from build123d import *

# Parameters (mm, degrees)
F0_W          = 4
F0_H          = 5
F0_R          = 3
F0_W_2        = 2
F0_H_2        = 8
F0_R_2        = 1.2
F1_DEPTH      = 10
F2_DEPTH      = 3
F3_START      = 2
F1_FACE_W     = 45
F1_FACE_H     = 20
F3_DEPTH      = 6.5
F4_START      = 5
F4_DEPTH      = 1.5
F5_R          = 5
F6_DEPTH      = 8.1
F7_DEPTH      = 3
F7_DEPTH_BACK = 0.5
F8_DEPTH      = 25
F8_DEPTH_BACK = 1.7
F10_START     = 16.22
F9_R          = 3.1
F10_DEPTH     = 9.58
F11_START     = 16.7
F9_R_2        = 1.15
F11_DEPTH     = 21.7


with BuildPart() as f1:
    # F0 (on Top) → F1 (new body)
    with BuildSketch(Plane.XY):
        Polygon((21.9938950613, 39.5450913161), (-23.0061049387, 39.5450913161), (-23.0061049387, 19.5450913161), (-9.9312635139, 19.5450913161), (10.0687364861, 19.5450913161), (21.9938950613, 19.5450913161), align=None)
        Polygon((-12.5061049387, 32.0450913161), (-12.5061049387, 37.0450913161), (19.4938950613, 37.0450913161), (19.4938950613, 22.0450913161), (-12.5061049387, 22.0450913161), (-12.5061049387, 27.0450913161), (-16.5061049387, 27.0450913161), (-20.5061049387, 27.0450913161), (-20.5061049387, 32.0450913161), (-16.5061049387, 32.0450913161), align=None, mode=Mode.SUBTRACT)
        with Locations((-18.5061049387, 29.5450913161)):
            Rectangle(F0_W, F0_H)
        with Locations((-14.5061049387, 29.5450913161)):
            Rectangle(F0_W, F0_H)
        Polygon((19.4938950613, 37.0450913161), (-12.5061049387, 37.0450913161), (-12.5061049387, 32.0450913161), (-12.5061049387, 27.0450913161), (-12.5061049387, 22.0450913161), (19.4938950613, 22.0450913161), align=None)
        with Locations((10.4938950613, 30.0450913161)):
            Circle(F0_R, mode=Mode.SUBTRACT)
        with Locations((17.2357911468, 31.5450913161)):
            Rectangle(F0_W_2, F0_H_2, mode=Mode.SUBTRACT)
        with Locations((10.4938950613, 30.0450913161)):
            Circle(F0_R)
        with Locations((10.4938950613, 30.0450913161)):
            Circle(F0_R_2, mode=Mode.SUBTRACT)
        with Locations((10.4938950613, 30.0450913161)):
            Circle(F0_R_2)
        with Locations((17.2357911468, 31.5450913161)):
            Rectangle(F0_W_2, F0_H_2)
    extrude(amount=F1_DEPTH)

    # F0 (on Top) → F2 (join)
    with BuildSketch(Plane.XY):
        Polygon((21.9938950613, 39.5450913161), (-23.0061049387, 39.5450913161), (-23.0061049387, 19.5450913161), (-9.9312635139, 19.5450913161), (10.0687364861, 19.5450913161), (21.9938950613, 19.5450913161), align=None)
        Polygon((-12.5061049387, 32.0450913161), (-12.5061049387, 37.0450913161), (19.4938950613, 37.0450913161), (19.4938950613, 22.0450913161), (-12.5061049387, 22.0450913161), (-12.5061049387, 27.0450913161), (-16.5061049387, 27.0450913161), (-20.5061049387, 27.0450913161), (-20.5061049387, 32.0450913161), (-16.5061049387, 32.0450913161), align=None, mode=Mode.SUBTRACT)
        with Locations((-14.5061049387, 29.5450913161)):
            Rectangle(F0_W, F0_H)
        with Locations((-18.5061049387, 29.5450913161)):
            Rectangle(F0_W, F0_H)
    extrude(amount=-F2_DEPTH)

    # F0 (on Top) + F1_face (on face) → F3 (cut)
    with BuildSketch(Plane.XY.offset(F3_START)):
        with Locations((-18.5061049387, 29.5450913161)):
            Rectangle(F0_W, F0_H)
        with Locations((-14.5061049387, 29.5450913161)):
            Rectangle(F0_W, F0_H)
    with BuildSketch(Plane(origin=(-0.5061049387, 29.5450913161, 10), x_dir=(1, 0, 0), z_dir=(0, 0, 1)).offset(F3_START)):
        Rectangle(F1_FACE_W, F1_FACE_H)
    extrude(amount=F3_DEPTH, mode=Mode.SUBTRACT)

    # F5
    f5_edges = [f1.edges().sort_by_distance(p)[0] for p in [
        (-23.006105, 39.545091, 3.5),
    ]]
    fillet(f5_edges, radius=F5_R)

    # F0 (on Top) → F6 (cut)
    with BuildSketch(Plane.XY):
        with Locations((10.4938950613, 30.0450913161)):
            Circle(F0_R_2)
    extrude(amount=F6_DEPTH, mode=Mode.SUBTRACT)



with BuildPart() as f4:
    # F0 (on Top) → F4 (new body)
    with BuildSketch(Plane.XY.offset(F4_START)):
        with Locations((10.4938950613, 30.0450913161)):
            Circle(F0_R)
        with Locations((10.4938950613, 30.0450913161)):
            Circle(F0_R_2, mode=Mode.SUBTRACT)
    extrude(amount=F4_DEPTH)


with BuildPart() as f1_1:
    add(f1.part)

    add(f4.part)  # F7 merges F4
    # F0 (on Top) → F7 (join, two sides)
    with BuildSketch(Plane.XY) as f7_sk:
        with Locations((10.4938950613, 30.0450913161)):
            Circle(F0_R)
        with Locations((10.4938950613, 30.0450913161)):
            Circle(F0_R_2, mode=Mode.SUBTRACT)
    extrude(amount=F7_DEPTH)
    extrude(f7_sk.sketch, amount=-F7_DEPTH_BACK)

    # F0 (on Top) → F8 (cut, two sides)
    with BuildSketch(Plane.XY) as f8_sk:
        with Locations((17.2357911468, 31.5450913161)):
            Rectangle(F0_W_2, F0_H_2)
    extrude(amount=-F8_DEPTH, mode=Mode.SUBTRACT)
    extrude(f8_sk.sketch, amount=F8_DEPTH_BACK, mode=Mode.SUBTRACT)

    # F9 (on Right) → F10 (cut)
    with BuildSketch(Plane.YZ.offset(F10_START)):
        with Locations((29.5450913161, 2)):
            Circle(F9_R)
    extrude(amount=F10_DEPTH, mode=Mode.SUBTRACT)

    # F9 (on Right) → F11 (cut)
    with BuildSketch(Plane.YZ.offset(F11_START)):
        with Locations((34.5450913161, 6)):
            Circle(F9_R_2)
        with Locations((24.595216945, 6)):
            Circle(F9_R_2)
    extrude(amount=F11_DEPTH, mode=Mode.SUBTRACT)


solid = f1_1.part
Input: part model. Units: mm. Frame: model coordinates. A direction names the side the tool comes from. Give positions to 0.01 mm unless a question says otherwise; leave off trailing zeros. Order: outer loops, then holes, each group sorted by start corner. A loop starts at its lowest first (then second) coordinate and runs counter-clockwise, first axis right, second up.
Q1. Draft query along X for faces 5 (the cylindrical face through (10.1, 33.02, -0.25)), 6 (the flat face through (-23.006, 27, 4)), 7 (the cylindrical face through (19.3, 33.4, 6.1)). Return one class per face: +X half, -X half, draft (parallel to the pull), parting line (faces both ways), or undercut.
Checked values:
face 5: undercut
face 6: -X half
face 7: draft
Q2. Contact query for flat-ended pins moving along their axis: pin 1 Ø10 at (x, y) = (-1.5, 32.5) entering from -Z; pin 2 Ø2.5 at (x, y) = (10, 29.5) entering from -Z; pin 3 Ø2 at (x, y) = (-7, 24.5) entering from -Z; pin 4 Ø1.4 at (x, y) = (10.49, 30.05) entering from -Z. Output: stop coordinate, or through.
Checked values:
pin 1: stops at z = -3
pin 2: stops at z = -0.5
pin 3: stops at z = 0
pin 4: stops at z = 8.1
Q3. Section D-D on z = 3.25. Output: boundary loops of the cut face in (x, y), and give its area (3 significant figures).
Checked values:
outline: (-23.01, 19.55) - (21.99, 19.55) - (21.99, 26.71) - (16.22, 26.71) - (16.22, 32.38) - (21.99, 32.38) - (21.99, 39.55) - (-18.01, 39.55) arc R5 ccw to (-23.01, 34.55) - close; hole (-20.51, 27.05) - (-12.51, 27.05) - (-12.51, 32.05) - (-20.51, 32.05) - close; hole circle Ø2.4 at (10.49, 30.05)
area: 817 mm2
Q4. Section B-B on z = -2. Output: boundary loops of the cut face in (x, y).
Checked values:
outline: (-23.01, 19.55) - (21.99, 19.55) - (21.99, 39.55) - (-18.01, 39.55) arc R5 ccw to (-23.01, 34.55) - close; hole (-12.51, 22.05) - (19.49, 22.05) - (19.49, 37.05) - (-12.51, 37.05) - close
Q5. Section C-C on y = 25.25. Output: boundary loops of the cut face in (x, z), and give its area (3 significant figures).
Checked values:
outline: (-23.01, -3) - (-12.51, -3) - (-12.51, 0) - (19.49, 0) - (19.49, -3) - (21.99, -3) - (21.99, 5.05) - (16.7, 5.05) - (16.7, 6.95) - (21.99, 6.95) - (21.99, 10) - (-23.01, 10) - close
area: 479 mm2
Q6. Section A-A on x = -5. Output: boundary loops of the cut face in (y, z), and give its area (3 significant figures).
Checked values:
outline: (19.55, -3) - (22.05, -3) - (22.05, 0) - (37.05, 0) - (37.05, -3) - (39.55, -3) - (39.55, 10) - (19.55, 10) - close
area: 215 mm2
Q7. Set-up query: faces 1 (the cylindrical face through (19.31, 23.446, 6.051)), 2 (the flat face through (19.494, 29.7, -1.5)), 3 (the flat face through (-16, 30, -3)), 4 (the flat face through (-20.506, 30, 5)). Return all of +Z, -Z, +X, -X, +Y, -Y with unobstructed straight access to the full face (end or side cutting, diameter ignored); none if empty.
Checked values:
face 1: +X
face 2: -Z
face 3: -Z, +X, -X, +Y, -Y
face 4: none
Q8. Ray query, probe 1 along X at (y, z) = (30, 3.5); probe 2 along Y at (x, z) = (20.6, 6); probe 3 along Y at (x, z) = (-18, 8). Return the intervals inside material, ascending.
Checked values:
probe 1: x = -23.01 to -20.51, -12.51 to 9.29, 11.69 to 16.22
probe 2: y = 19.55 to 23.45, 25.75 to 33.4, 35.7 to 39.55
probe 3: y = 19.55 to 27.05, 32.05 to 39.55
